```python
from build123d import *

# Parameters (mm, degrees)
F0_W     = 35
F0_H     = 50
F1_DEPTH = 650
F2_SIZE  = 6
F3_SIZE  = 4
F4_SIZE  = 2
F5_SIZE  = 2


with BuildPart() as f1:
    # F0 (on Top) → F1 (new body)
    with BuildSketch(Plane.XY):
        Rectangle(F0_W, F0_H)
    extrude(amount=F1_DEPTH)

    # F2
    f2_edges = [f1.edges().sort_by_distance(p)[0] for p in [
        (-17.5, 25, 325),
        (17.5, 25, 325),
    ]]
    chamfer(f2_edges, length=F2_SIZE)

    # F3
    f3_edges = [f1.edges().sort_by_distance(p)[0] for p in [
        (-17.5, 19, 325),
        (17.5, 19, 325),
    ]]
    chamfer(f3_edges, length=F3_SIZE)

    # F4
    f4_edges = [f1.edges().sort_by_distance(p)[0] for p in [
        (-11.5, 25, 325),
        (11.5, 25, 325),
    ]]
    chamfer(f4_edges, length=F4_SIZE)

    # F5
    f5_edges = [f1.edges().sort_by_distance(p)[0] for p in [
        (-17.5, 15, 325),
        (17.5, 15, 325),
    ]]
    chamfer(f5_edges, length=F5_SIZE)


solid = f1.part
```
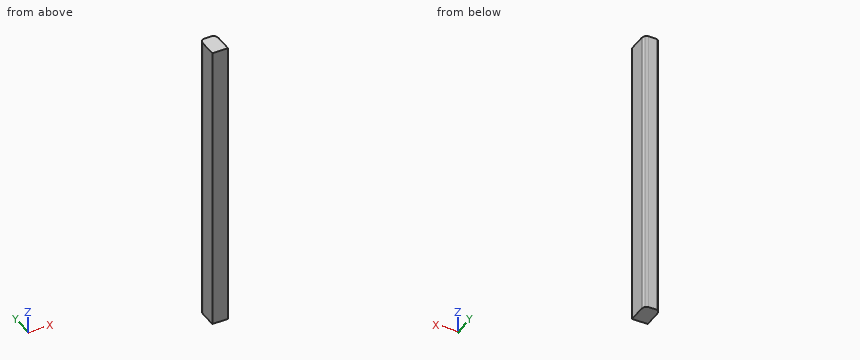
Could you check a few things on this model? Use its own coordinates, in mm. Round coordinates to 2 decimals unless told otherwise and drop trailing zeros. Loops run counter-clockwise (first coordinate to the right, second up) from the corner with the lowest first, then second, coordinate; pieces in that order, holes last. Notation, with made-up numbers: (73.5, -29) - (125.5, -29) arc R15 cw to (125.5, -21) - close; hole circle Ø5 at (22, -31). An arc over 180 degrees is marked (long way). Answer as CSV lines item,"result".
1. For pin 1 Ø1 at (x, z) = (-10.5, 338) entering from +Y, with a flat end and sliding along its axis, tell me the tip position at first contact or that it passes through.
Filled in:
pin 1,"stops at y = 24.79"
2. I want a section at A-A on z = 272.5. List the corners of the cut face in (x, y) for me.
Filled in:
outline,"(-17.5, -25) - (17.5, -25) - (17.5, 13) - (16.73, 16.85) - (14.67, 21.83) - (12.91, 23.59) - (9.5, 25) - (-9.5, 25) - (-12.91, 23.59) - (-14.67, 21.83) - (-16.73, 16.85) - (-17.5, 13) - close"
3. Please list where these lines run through material, in increasing order: line 1 along Y through (x, z) = (-14.5, 311); line 2 along Y through (x, z) = (15.5, 80.5); line 3 along X through (y, z) = (23.5, 306.5). Write a range as [from, to].
Filled in:
line 1,"y = [-25, 22]"
line 2,"y = [-25, 19.83]"
line 3,"x = [-13, 13]"
